Input: dimensioned drawing with shaded views. Units: mm. Origin: part minimum x, y, z. A direction names the side the tool comes from. Coordinates: 2 decimals unless noted, no trailing zeros. Order: outer loops, then holes, each group sorted by start corner. A loop starts at its lowest first (then second) coordinate and runs counter-clockwise, first axis right, second up.
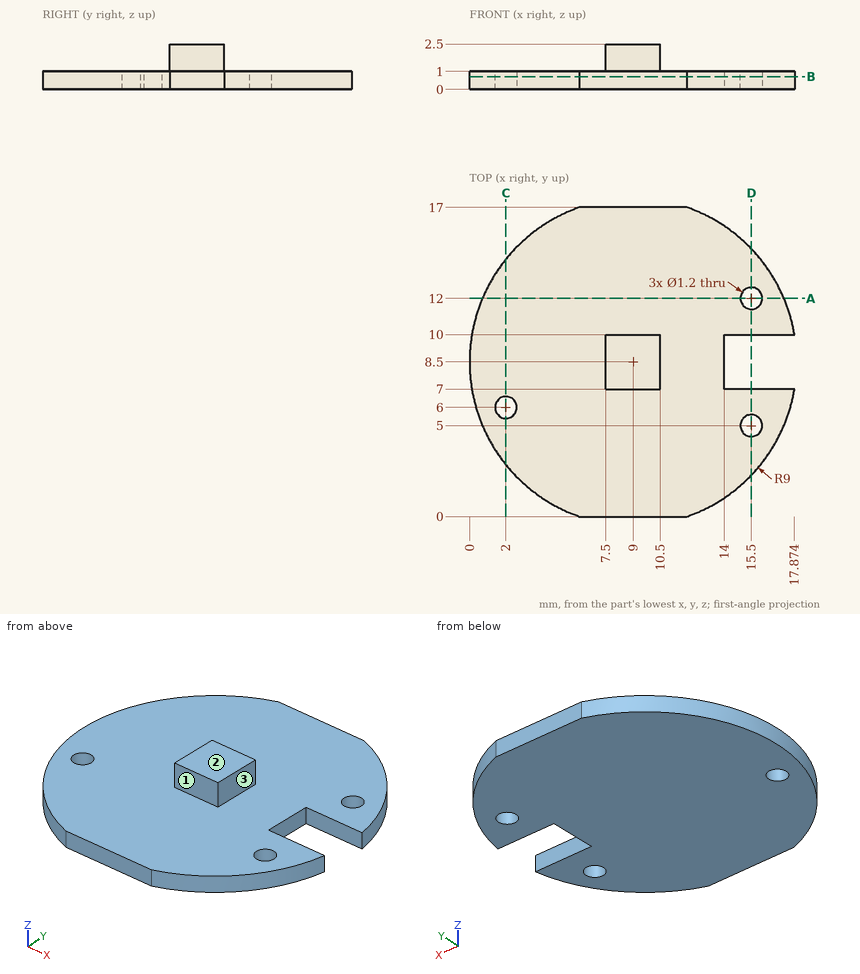
1. Contact query for flat-ended pins moving along their axis: P1, Ø1.1, axis at y = 8.5, z = 0.5, coming from the +X side; P2, Ø1.6, axis at x = 15.5, y = 5, coming from the +Z side; P3, Ø0.5, axis at x = 16.5, z = 0.5, coming from the -Y side; P4, Ø3, axis at x = 11, y = 6, coming from the +Z side. Output: stop coordinate, or through.
2. Section query B-B, the plane z = 0.7. Output: boundary loops of the cut face in (x, y), plus the area to 3 significant figures.
3. Access query for the marked faces 1, 2 and 3. Directions: +Z, -Z, +X, -X, +Y, -Y. A direction counts if a zero-diameter tool reaches every point of the face in a straight line with its end or side. Return the directions, or none.
4. Section query D-D, the plane x = 15.5. Output: boundary loops of the cut face in (y, z) (3 decimals).
5. Material intervals for line 1 along Y through (x, z) = (15.5, 0.85) (1 decimal); line 2 along Z through (x, y) = (2.5, 7.5); line 3 along Y through (x, z) = (10, 1.55), sorted ascending.
6. Section query C-C, the plane x = 2. Output: boundary loops of the cut face in (y, z).
7. Section query A-A, the plane y = 12. Output: boundary loops of the cut face in (x, z), plus the area to 3 significant figures.
Answer key:
1. P1: stops at x = 14
1. P2: stops at z = 1
1. P3: stops at y = 3.17
1. P4: stops at z = 2.5
2. outline: (6.04, 0) - (11.96, 0) arc R9 ccw to (17.87, 7) - (14, 7) - (14, 10) - (17.87, 10) arc R9 ccw to (11.96, 17) - (6.04, 17) arc R9 ccw to start; hole circle Ø1.2 at (2, 6); hole circle Ø1.2 at (15.5, 5); hole circle Ø1.2 at (15.5, 12)
2. area: 235 mm2
3. face 1: +Z, +X, -X, -Y
3. face 2: +Z, +X, -X, +Y, -Y
3. face 3: +Z, +X, +Y, -Y
4. outline: (2.275, 0) - (4.4, 0) - (4.4, 1) - (2.275, 1) - close; (5.6, 0) - (7, 0) - (7, 1) - (5.6, 1) - close; (10, 0) - (11.4, 0) - (11.4, 1) - (10, 1) - close; (12.6, 0) - (14.725, 0) - (14.725, 1) - (12.6, 1) - close
5. line 1: y = 2.3 to 4.4, 5.6 to 7, 10 to 11.4, 12.6 to 14.7
5. line 2: z = 0 to 1
5. line 3: y = 7 to 10
6. outline: (2.84, 0) - (5.4, 0) - (5.4, 1) - (2.84, 1) - close; (6.6, 0) - (14.16, 0) - (14.16, 1) - (6.6, 1) - close
7. outline: (0.71, 0) - (14.9, 0) - (14.9, 1) - (0.71, 1) - close; (16.1, 0) - (17.29, 0) - (17.29, 1) - (16.1, 1) - close
7. area: 15.4 mm2
